```python
from build123d import *

# Parameters (mm, degrees)
SKETCH2_W           = 33.15
SKETCH2_H           = 33
BOSS_EXTRUDE1_DEPTH = 7.5
SKETCH3_R           = 1.175
CUT_EXTRUDE1_DEPTH  = 4.5
SKETCH4_W           = 5.3
SKETCH4_H           = 7
CUT_EXTRUDE2_DEPTH  = 3.5
SKETCH5_W           = 17.312690108
SKETCH5_H           = 1.808425299
CUT_EXTRUDE3_DEPTH  = 2
SKETCH6_W           = 5.3
SKETCH6_H           = 3.3
CUT_EXTRUDE4_DEPTH  = 25.560753755
CHAMFER3_SIZE       = 11
CHAMFER3_SIZE2      = 6.350852961
SKETCH7_W           = 3
SKETCH7_H           = 33
SKETCH7_H_2         = 30
BOSS_EXTRUDE2_DEPTH = 30
SKETCH8_W           = 33.15
SKETCH8_H           = 37.5
BOSS_EXTRUDE3_DEPTH = 1
SKETCH9_W           = 1.5
SKETCH9_H           = 2
CUT_EXTRUDE5_DEPTH  = 31.5
SKETCH10_W          = 27.15
SKETCH10_H          = 2
CUT_EXTRUDE6_DEPTH  = 1.5
CUT_EXTRUDE7_START  = -30
SKETCH11_W          = 1.5
SKETCH11_H          = 2
CUT_EXTRUDE7_DEPTH  = 30
SKETCH14_W          = 30.15
SKETCH14_H          = 2
CUT_EXTRUDE8_DEPTH  = 1.5


with BuildPart() as part:
    # Sketch2 → Boss-Extrude1 (new body)
    with BuildSketch(Plane.XY):
        Rectangle(SKETCH2_W, SKETCH2_H)
    extrude(amount=BOSS_EXTRUDE1_DEPTH)

    # Sketch3 → Cut-Extrude1 (cut)
    with BuildSketch(Plane.XY):
        with Locations((10.325, 10.25)):
            Circle(SKETCH3_R)
        with Locations((-10.325, 10.25)):
            Circle(SKETCH3_R)
        with Locations((10.325, -10.25)):
            Circle(SKETCH3_R)
        with Locations((-10.325, -10.25)):
            Circle(SKETCH3_R)
    extrude(amount=CUT_EXTRUDE1_DEPTH, mode=Mode.SUBTRACT)

    # Sketch4 → Cut-Extrude2 (cut)
    with BuildSketch(Plane.XY):
        with Locations((9.775, 0)):
            Rectangle(SKETCH4_W, SKETCH4_H)
        with Locations((-9.775, 0)):
            Rectangle(SKETCH4_W, SKETCH4_H)
    extrude(amount=CUT_EXTRUDE2_DEPTH, mode=Mode.SUBTRACT)

    # Sketch5 → Cut-Extrude3 (cut)
    with BuildSketch(Plane.XY):
        with Locations((-0.109621432, -11.80915301)):
            Rectangle(SKETCH5_W, SKETCH5_H)
    extrude(amount=CUT_EXTRUDE3_DEPTH, mode=Mode.SUBTRACT)

    # Sketch6 → Cut-Extrude4 (cut, through all)
    with BuildSketch(Plane.XY):
        Rectangle(SKETCH6_W, SKETCH6_H)
    extrude(amount=CUT_EXTRUDE4_DEPTH, mode=Mode.SUBTRACT)

    # Chamfer3
    chamfer3_edges = [part.edges().sort_by_distance(p)[0] for p in [
        (2.65, 0, 7.5),
        (0, 1.65, 7.5),
        (-2.65, 0, 7.5),
        (0, -1.65, 7.5),
    ]]
    chamfer3_side = [part.faces().sort_by_distance(p)[0] for p in [
        (-16.107247662, 0, 7.5),
    ]]
    chamfer(chamfer3_edges, length=CHAMFER3_SIZE, length2=CHAMFER3_SIZE2, reference=chamfer3_side[0])

    # Sketch7 → Boss-Extrude2 (add)
    with BuildSketch(Plane.XY):
        with Locations((15.075, 0)):
            Rectangle(SKETCH7_W, SKETCH7_H)
        Polygon((-13.575, 13.5), (13.575, 13.5), (13.575, 16.5), (-16.575, 16.5), (-16.575, 13.5), align=None)
        with Locations((-15.075, -1.5)):
            Rectangle(SKETCH7_W, SKETCH7_H_2)
    extrude(amount=-BOSS_EXTRUDE2_DEPTH)

    # Sketch8 → Boss-Extrude3 (add)
    with BuildSketch(Plane(origin=(0, 16.5, 0), x_dir=(1, 0, 0), z_dir=(0, 1, 0))):
        with Locations((0, 11.25)):
            Rectangle(SKETCH8_W, SKETCH8_H)
    extrude(amount=BOSS_EXTRUDE3_DEPTH)

    # Sketch9 → Cut-Extrude5 (cut)
    with BuildSketch(Plane.XZ.offset(16.5)):
        with Locations((-14.325, -27)):
            Rectangle(SKETCH9_W, SKETCH9_H)
        with Locations((14.325, -27)):
            Rectangle(SKETCH9_W, SKETCH9_H)
    extrude(amount=-CUT_EXTRUDE5_DEPTH, mode=Mode.SUBTRACT)

    # Sketch10 → Cut-Extrude6 (cut)
    with BuildSketch(Plane.XZ.offset(-13.5)):
        with Locations((0, -27)):
            Rectangle(SKETCH10_W, SKETCH10_H)
    extrude(amount=-CUT_EXTRUDE6_DEPTH, mode=Mode.SUBTRACT)

    # Sketch11 → Cut-Extrude7 (cut)
    with BuildSketch(Plane(origin=(0, 0, -30), x_dir=(-1, 0, 0), z_dir=(0, 0, -1)).offset(CUT_EXTRUDE7_START)):
        with Locations((-14.325, -14)):
            Rectangle(SKETCH11_W, SKETCH11_H)
        with Locations((14.325, -14)):
            Rectangle(SKETCH11_W, SKETCH11_H)
    extrude(amount=CUT_EXTRUDE7_DEPTH, mode=Mode.SUBTRACT)

    # Sketch14 → Cut-Extrude8 (cut)
    with BuildSketch(Plane(origin=(0, 0, 0), x_dir=(-1, 0, 0), z_dir=(0, 0, -1))):
        with Locations((0, -14)):
            Rectangle(SKETCH14_W, SKETCH14_H)
    extrude(amount=-CUT_EXTRUDE8_DEPTH, mode=Mode.SUBTRACT)


solid = part.part
```
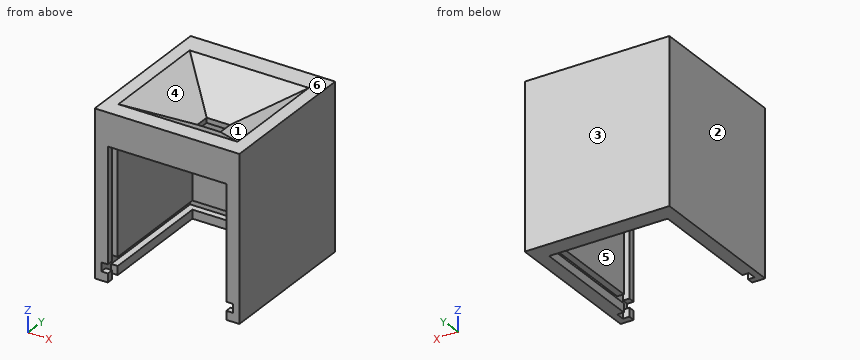
Geometry: final body of the model. Coordinates: model frame, mm. Face numbers are marked on the shaded views. A direction names the side the tool comes from. Coordinates: 2 decimals unless noted, no trailing zeros. Order: outer loops, then holes, each group sorted by start corner. A loop starts at its lowest first (then second) coordinate and runs counter-clockwise, first axis right, second up. Notation, with made-up numbers: (-29, -40) - (4, -40) arc R10 cw to (4, -31) - close; hole circle Ø11 at (4, 31.25). An arc over 180 degrees is marked (long way). Return JSON: item names as keys, results as strings. Group by question number.
1. Set-up query: the marked faces 4, 5 and 6. Return all of +Z, -Z, +X, -X, +Y, -Y with unobstructed straight access to the full face (end or side cutting, diameter ignored); none if empty.
2. Cut plane B-B (z = -14.5). Output: boundary loops of the cut face in (x, y) (3 decimals), plus the area to 3 significant figures.
3. Cut plane C-C (y = 14). Output: boundary loops of the cut face in (x, z) (3 decimals).
4. Cut plane D-D (x = -6). Output: boundary loops of the cut face in (y, z), plus the area to 3 significant figures.
5. Pin query (flat end, axial travel): pin 1 (8.5 mm diameter, centred on x = 5, y = -2, fed in from +Z); pin 2 (13 mm diameter, centred on x = 2, z = -9.5, fed in from -Y); pin 3 (2.5 mm diameter, centred on x = -10.325, y = 10.25, fed in from -Z). Return the tip coordinate at first contact, or that it passes through.
6. Material intervals for line 1 along Y through (x, z) = (-14.5, -16.5); line 2 along X through (y, z) = (4.5, -21) (3 decimals); line 3 along X through (y, z) = (-10, 3) (3 decimals), sorted ascending. Write a range as [from, to].
7. Pull-direction query (Y, two-part tool) for the marked faces 1, 2 and 3; classes: pulls with the +Y half, pulls with the -Y half, needs draft (parallel to the pull), parting line crosses it, or undercut.
8. Cut plane A-A (x = 14.5). Output: boundary loops of the cut face in (y, z).
Resolved:
{
 "1": {"face 4": "+Z", "face 5": "-Z, -Y", "face 6": "+Z, +X, -X, +Y, -Y"},
 "2": {"outline": "(-16.575, -16.5) - (-13.575, -16.5) - (-13.575, -15) - (-15.075, -15) - (-15.075, -13) - (-13.575, -13) - (-13.575, 13.5) - (13.575, 13.5) - (13.575, -13) - (15.075, -13) - (15.075, -15) - (13.575, -15) - (13.575, -16.5) - (16.575, -16.5) - (16.575, 17.5) - (-16.575, 17.5) - close", "area": "307 mm²"},
 "3": {"outline": "(-16.575, -30) - (16.575, -30) - (16.575, 7.5) - (-16.575, 7.5) - close; hole (-15.075, -28) - (15.075, -28) - (15.075, -26) - (-15.075, -26) - close"},
 "4": {"outline": "(-16.5, 0) - (-15, 0) - (-15, 1.5) - (-13, 1.5) - (-13, 0) - (-12.71, 0) - (-12.71, 2) - (-10.9, 2) - (-10.9, 0) - (13.5, 0) - (13.5, -26) - (15, -26) - (15, -28) - (13.5, -28) - (13.5, -30) - (17.5, -30) - (17.5, 7.5) - (12.65, 7.5) - (5, 3.08) - (-5, 3.08) - (-12.65, 7.5) - (-16.5, 7.5) - close", "area": "287 mm²"},
 "5": {"pin 1": "stops at z = 4.96", "pin 2": "stops at y = 13.5", "pin 3": "stops at z = 0"},
 "6": {"line 1": "y = [-16.5, -15], [-13, 17.5]", "line 2": "x = [-16.575, -13.575], [13.575, 16.575]", "line 3": "x = [-16.575, -11.473], [-9.177, 9.177], [11.473, 16.575]"},
 "7": {"face 1": "undercut", "face 2": "needs draft", "face 3": "pulls with the +Y half"},
 "8": {"outline": "(-16.5, -30) - (-15, -30) - (-15, -28) - (-16.5, -28) - close; (-16.5, -26) - (-15, -26) - (-15, 1.5) - (-13, 1.5) - (-13, -26) - (15, -26) - (15, -28) - (-13, -28) - (-13, -30) - (17.5, -30) - (17.5, 7.5) - (-16.5, 7.5) - close"}
}
